Read the model definition and answer for the solid it produces. Units are mm, in the model's axes. A direction names the side the tool comes from. Give positions to 0.01 mm unless a question says otherwise; leave off trailing zeros. Write each loop counter-clockwise with the first axis right and the second up, starting at its lowest first coordinate (ties: lowest second). Pieces come first, ordered by that corner, then holes. Notation, with made-up numbers: M 73,41 L 100,41 A32 ccw 100,69 Z; hole C 33.5,47.25 d1. An arc over 180 degrees is marked long. Write each question's results on one line, items separated by ' | '. Start each with the question number.
```python
from build123d import *

# Parameters (mm, degrees)
SKETCH1_W                 = 1.5
SKETCH1_H                 = 1.5
BASE_BLOCK_DEPTH          = 1
SKETCH2_W                 = 4.8
SKETCH2_H                 = 0.75
BASE_BRIDGE_DEPTH         = 1.5
LOWER_SIDE_1_DEPTH        = 1.45
SKETCH6_R                 = 1
PIVOT_DEPTH               = 1
BODY_BLOCK_DEPTH          = 3.7
SKETCH8_W                 = 1.9
SKETCH8_H                 = 8.25
REAR_CUT_THROUGH_DEPTH    = 24.222672112
CLIP_FORMING_DEPTH        = 2.75
THROUGH_HOLES_DEPTH       = 23.941501695
SKETCH11_W                = 1.9
SKETCH11_H                = 7.5
PCB_SLOT_DEPTH            = 4.95
THROUGH_HOLE_REAR_1_DEPTH = 1.023508356
THROUGH_HOLE_REAR_2_DEPTH = 1.023508356
SKETCH15_W                = 1.9
SKETCH15_H                = 1.3
PCB_SLOT_TOP_DEPTH        = 0.25
REAR_FILLET_2MM_R         = 2
REAR_FILLET_1MM_R         = 1
GUIDE_FILLET_0_25MM_R     = 0.25
GUIDE_FILLET_0_5MM_R      = 0.5


# Some blends are built 0.0001 mm under size
with BuildPart() as part:
    # Sketch1 → Base Block (new body)
    with BuildSketch(Plane(origin=(0, 0, 0), x_dir=(1, 0, 0), z_dir=(0, 1, 0))):
        Rectangle(SKETCH1_W, SKETCH1_H)
    extrude(amount=BASE_BLOCK_DEPTH)

    # Sketch2 → Base Bridge (add)
    with BuildSketch(Plane.ZY.offset(0.75)):
        with Locations((0, 0.375)):
            Rectangle(SKETCH2_W, SKETCH2_H)
    extrude(amount=BASE_BRIDGE_DEPTH)

    # Sketch5 → Lower Side 1 (add)
    with BuildSketch(Plane.XY.offset(2.4)):
        with BuildLine():
            Line((-0.75, 0), (-2.75, 0))
            Line((-2.75, 0), (-2.75, 1.75))
            Line((-2.75, 1.75), (-4.917566413, 3.413326741))
            ThreePointArc((-4.917566413, 3.413326741), (-5.493757624, 4.115447239), (-5.7, 5))
            Line((-5.7, 5), (-5.7, 14))
            Line((-5.7, 14), (-8.35, 16.15))
            Line((-8.35, 16.15), (-8.35, 21.3))
            ThreePointArc((-8.35, 21.3), (-7.65, 22), (-6.95, 21.3))
            Line((-6.95, 21.3), (-6.95, 18.8))
            Line((-6.95, 18.8), (0.25, 18.8))
            Line((0.25, 18.8), (0.25, 15.2))
            Line((0.25, 15.2), (-3, 15.2))
            Line((-3, 15.2), (-3, 12.45))
            Line((-3, 12.45), (-0.2, 12.45))
            Line((-0.2, 12.45), (-0.2, 9.7))
            Line((-0.2, 9.7), (-3, 9.7))
            Line((-3, 9.7), (-3, 8.7))
            ThreePointArc((-3, 8.7), (-2.725432986, 7.572457553), (-1.963210212, 6.697383009))
            ThreePointArc((-1.963210212, 6.697383009), (-0.621213938, 4.811248727), (-0.75, 2.5))
            Line((-0.75, 2.5), (-0.853553391, 2.25))
            Line((-0.853553391, 2.25), (-0.75, 2))
            Line((-0.75, 2), (-0.75, 0))
        make_face()
    lower_side_1 = extrude(amount=-LOWER_SIDE_1_DEPTH)

    # Sketch6 → Pivot (add)
    with BuildSketch(Plane.XY.offset(2.4)):
        with Locations(Location((-3.7, 5, 0), (0, 0, 180))):
            Circle(SKETCH6_R)
    pivot = extrude(amount=PIVOT_DEPTH)

    # Lower Side 2: Lower Side 1, Pivot across plane
    add(lower_side_1.mirror(Plane.XY))
    add(pivot.mirror(Plane.XY))

    # Sketch7 → Body Block (add, symmetric)
    with BuildSketch(Plane.XY):
        with BuildLine():
            Line((-8.35, 16.15), (-5.7, 14))
            Line((-5.7, 14), (-5.7, 7.95))
            Line((-5.7, 7.95), (-5.2, 7.95))
            Line((-5.2, 7.95), (-3.9, 9.2))
            Line((-3.9, 9.2), (-3, 9.2))
            Line((-3, 9.2), (-3, 9.7))
            Line((-3, 9.7), (-0.2, 9.7))
            Line((-0.2, 9.7), (-0.2, 12.45))
            Line((-0.2, 12.45), (-3, 12.45))
            Line((-3, 12.45), (-3, 15.2))
            Line((-3, 15.2), (0.25, 15.2))
            Line((0.25, 15.2), (0.25, 18.8))
            Line((0.25, 18.8), (-4.95, 18.8))
            Line((-4.95, 18.8), (-4.95, 19.25))
            Line((-4.95, 19.25), (-5.45, 19.25))
            Line((-5.45, 19.25), (-5.45, 19.75))
            Line((-5.45, 19.75), (-5.95, 19.75))
            Line((-5.95, 19.75), (-5.95, 20.25))
            Line((-5.95, 20.25), (-6.45, 20.25))
            Line((-6.45, 20.25), (-6.45, 20.75))
            Line((-6.45, 20.75), (-6.95, 20.75))
            Line((-6.95, 20.75), (-6.95, 21.3))
            ThreePointArc((-6.95, 21.3), (-7.65, 22), (-8.35, 21.3))
            Line((-8.35, 21.3), (-8.35, 16.15))
        make_face()
    extrude(amount=BODY_BLOCK_DEPTH, both=True)

    # Sketch8 → Rear Cut Through (cut, through all)
    with BuildSketch(Plane.ZY.offset(5.7)):
        with Locations((0, 5.875)):
            Rectangle(SKETCH8_W, SKETCH8_H)
    extrude(amount=-REAR_CUT_THROUGH_DEPTH, mode=Mode.SUBTRACT)

    # Sketch9 → Clip Forming (cut)
    with BuildSketch(Plane(origin=(0, 12.45, 0), x_dir=(1, 0, 0), z_dir=(0, 1, 0))):
        with BuildLine():
            Line((-1.3, -2.2), (-0.406587956, -2.357532648))
            ThreePointArc((-0.406587956, -2.357532648), (-0.258488889, -2.443037684), (-0.2, -2.603734587))
            Line((-0.2, -2.603734587), (-0.2, 2.603734587))
            ThreePointArc((-0.2, 2.603734587), (-0.258488889, 2.443037684), (-0.406587956, 2.357532648))
            Line((-0.406587956, 2.357532648), (-1.3, 2.2))
            Line((-1.3, 2.2), (-1.3, 2.55))
            Line((-1.3, 2.55), (-3, 2.55))
            Line((-3, 2.55), (-3, -2.55))
            Line((-3, -2.55), (-1.3, -2.55))
            Line((-1.3, -2.55), (-1.3, -2.2))
        make_face()
    extrude(amount=-CLIP_FORMING_DEPTH, mode=Mode.SUBTRACT)

    # Sketch10 → Through Holes (cut, through all)
    with BuildSketch(Plane(origin=(-3, 0, 0), x_dir=(0, 0, -1), z_dir=(1, 0, 0))):
        Polygon((-2.55, 14.45), (-1.526491644, 14.45), (-1.526491644, 9.95), (-2.026491644, 9.45), (-2.55, 9.45), align=None)
        Polygon((2.55, 14.45), (2.55, 9.45), (2.026491644, 9.45), (1.526491644, 9.95), (1.526491644, 14.45), align=None)
    extrude(amount=-THROUGH_HOLES_DEPTH, mode=Mode.SUBTRACT)

    # Sketch11 → PCB Slot (cut)
    with BuildSketch(Plane(origin=(0.25, 0, 0), x_dir=(0, 0, -1), z_dir=(1, 0, 0))):
        with Locations((0, 13.75)):
            Rectangle(SKETCH11_W, SKETCH11_H)
    extrude(amount=-PCB_SLOT_DEPTH, mode=Mode.SUBTRACT)

    # Sketch13 → Through Hole Rear 1 (cut)
    with BuildSketch(Plane.XY.offset(-2.55)):
        Polygon((-8.35, 20.2), (-4, 16.5), (-4, 14.45), (-6.254651163, 14.45), (-8.35, 16.15), align=None)
    extrude(amount=THROUGH_HOLE_REAR_1_DEPTH, mode=Mode.SUBTRACT)

    # Sketch14 → Through Hole Rear 2 (cut)
    with BuildSketch(Plane(origin=(0, 0, 2.55), x_dir=(-1, 0, 0), z_dir=(0, 0, -1))):
        Polygon((8.35, 20.2), (4, 16.5), (4, 14.45), (6.254651163, 14.45), (8.35, 16.15), align=None)
    extrude(amount=THROUGH_HOLE_REAR_2_DEPTH, mode=Mode.SUBTRACT)

    # Sketch15 → PCB Slot Top (cut)
    with BuildSketch(Plane(origin=(0.25, 0, 0), x_dir=(0, 0, -1), z_dir=(1, 0, 0))):
        with Locations((0, 18.15)):
            Rectangle(SKETCH15_W, SKETCH15_H)
    extrude(amount=-PCB_SLOT_TOP_DEPTH, mode=Mode.SUBTRACT)

    # Rear Fillet (2mm)
    rear_fillet_2mm_edges = [part.edges().sort_by_distance(p)[0] for p in [
        (-5.7, 14, 3.125),
        (-5.7, 14, 0),
        (-5.7, 14, -3.125),
    ]]
    fillet(rear_fillet_2mm_edges, radius=REAR_FILLET_2MM_R)

    # Rear Fillet (1mm)
    rear_fillet_1mm_edges = [part.edges().sort_by_distance(p)[0] for p in [
        (-8.35, 16.15, 0),
        (-8.35, 16.15, -3.125),
        (-8.35, 16.15, 3.125),
    ]]
    fillet(rear_fillet_1mm_edges, radius=REAR_FILLET_1MM_R)

    # Guide Fillet (0.25mm)
    guide_fillet_0_25mm_edges = [part.edges().sort_by_distance(p)[0] for p in [
        (0.25, 17, -0.95),
        (0.25, 17, 0.95),
        (0.25, 18.8, -2.325),
        (0.25, 18.8, 2.325),
    ]]
    fillet(guide_fillet_0_25mm_edges, radius=GUIDE_FILLET_0_25MM_R - 0.0001)  # a hair under: the kernel refuses the full size

    # Guide Fillet (0.5mm)
    # the kernel refuses this fillet: 0.5 mm, written as the material it takes off along each edge
    with BuildSketch(Plane(origin=(0.25, 15.2, -4.95), x_dir=(-1, 0, 0), z_dir=(0, 0, 1))) as guide_fillet_0_5mm_piece_1:
        with BuildLine():
            CenterArc((GUIDE_FILLET_0_5MM_R, -GUIDE_FILLET_0_5MM_R), GUIDE_FILLET_0_5MM_R, 90, 90)
            Line((0, -GUIDE_FILLET_0_5MM_R), (0, 0))
            Line((0, 0), (GUIDE_FILLET_0_5MM_R, 0))
        make_face()
    extrude(amount=5.0001, mode=Mode.SUBTRACT)
    with BuildSketch(Plane(origin=(0.25, 15.2, -0.0501), x_dir=(0, 1, 0), z_dir=(0, 0, 1))) as guide_fillet_0_5mm_piece_2:
        with BuildLine():
            CenterArc((GUIDE_FILLET_0_5MM_R, GUIDE_FILLET_0_5MM_R), GUIDE_FILLET_0_5MM_R, 180, 90)
            Line((0, GUIDE_FILLET_0_5MM_R), (0, 0))
            Line((0, 0), (GUIDE_FILLET_0_5MM_R, 0))
        make_face()
    extrude(amount=5.0001, mode=Mode.SUBTRACT)


solid = part.part
```
Item 1: For faces 4 (the flat face through (-3.5, 14.45, 2)), 5 (the flat face through (-4.559, 8.566, -3.041)), 6 (the flat face through (-2.75, 1, 2)), determine the directions among +Z, -Z, +X, -X, +Y, -Y from which every point of the face is accessible in a straight line to the end or side of a thin tool.
Item 2: Section C-C, the plane x = -4.5 is taken. Give the number of separate pieces and of enclosed holes in the cut face, then the cut area to 3 significant figures.
Item 3: Section B-B, the plane y = 12.75 is taken. Determine the outline of the cut face in (x, z), then the cut area to 3 significant figures.
Item 4: Straight lines are drawn through the part: line 1 (Z direction, x = -7.5, y = 16.75); line 2 (Z direction, x = -3.25, y = 7.25); line 3 (Z direction, x = -2, y = 17.25). For each, find the intervals that lie inside material, in ascending order.
Item 5: Section A-A, the plane z = 0.5 is taken. Determine the outline of the cut face in (x, y).
Item 6: Section D-D, the plane y = 3 is taken. Determine the outline of the cut face in (x, z), then the cut area to 3 significant figures.
Item 7: Given P1, Ø1, axis at x = -5, z = 0.5, coming from the +Y side; P2, Ø0.8, axis at x = -5.5, z = 0, coming from the -Y side; P3, Ø1.5, axis at x = -5, y = 4, coming from the +Z side, each flat-ended and moving along its own axis, determine where each tip first touches the part or whether it passes through.
Item 8: Determine the mould class of faces 1 (the flat face through (0, 0.5, -0.75)), 2 (the flat face through (-5, 10, 0)), 3 (the flat face through (-3, 7, -0.95)) for opening direction Y: +Y half, -Y half, draft (parallel to the pull), parting line (faces both ways), or undercut.
Worked out:
1) face 4: +X, -X | face 5: -Z, +X | face 6: +Z, -Z, -X, -Y
2) separate pieces: 1 | enclosed holes: 2 | area: 61.8 mm²
3) outline: M -5.7,-3.7 L -3,-3.7 L -3,-2.55 L -5.7,-2.55 Z; M -5.7,-1.53 L -3,-1.53 L -3,-0.95 L -4.7,-0.95 L -4.7,0.95 L -3,0.95 L -3,1.53 L -5.7,1.53 Z; M -5.7,2.55 L -3,2.55 L -3,3.7 L -5.7,3.7 Z | area: 11.2 mm²
4) line 1: z = -3.7 to -2.55, -1.53 to 1.53, 2.55 to 3.7 | line 2: z = -2.4 to -0.95, 0.95 to 2.4 | line 3: z = -3.7 to -0.95, 0.95 to 3.7
5) outline: M -8.35,16.63 A1 ccw -7.98,15.85 L -6.44,14.6 A2 cw -5.7,13.05 L -5.7,10 L -4.7,10 L -4.7,17.5 L 0,17.5 L 0,18.8 L -4.95,18.8 L -4.95,19.25 L -5.45,19.25 L -5.45,19.75 L -5.95,19.75 L -5.95,20.25 L -6.45,20.25 L -6.45,20.75 L -6.95,20.75 L -6.95,21.3 A0.7 ccw -8.35,21.3 Z; M -2.25,0 L 0.75,0 L 0.75,1 L -0.75,1 L -0.75,0.75 L -2.25,0.75 Z
6) outline: M -4.38,-2.4 L -0.59,-2.4 L -0.59,-0.95 L -4.38,-0.95 Z; M -4.38,0.95 L -0.59,0.95 L -0.59,2.4 L -4.38,2.4 Z | area: 11.0 mm²
7) P1: stops at y = 19.75 | P2: stops at y = 10 | P3: stops at z = 3.4
8) face 1: draft | face 2: -Y half | face 3: undercut
